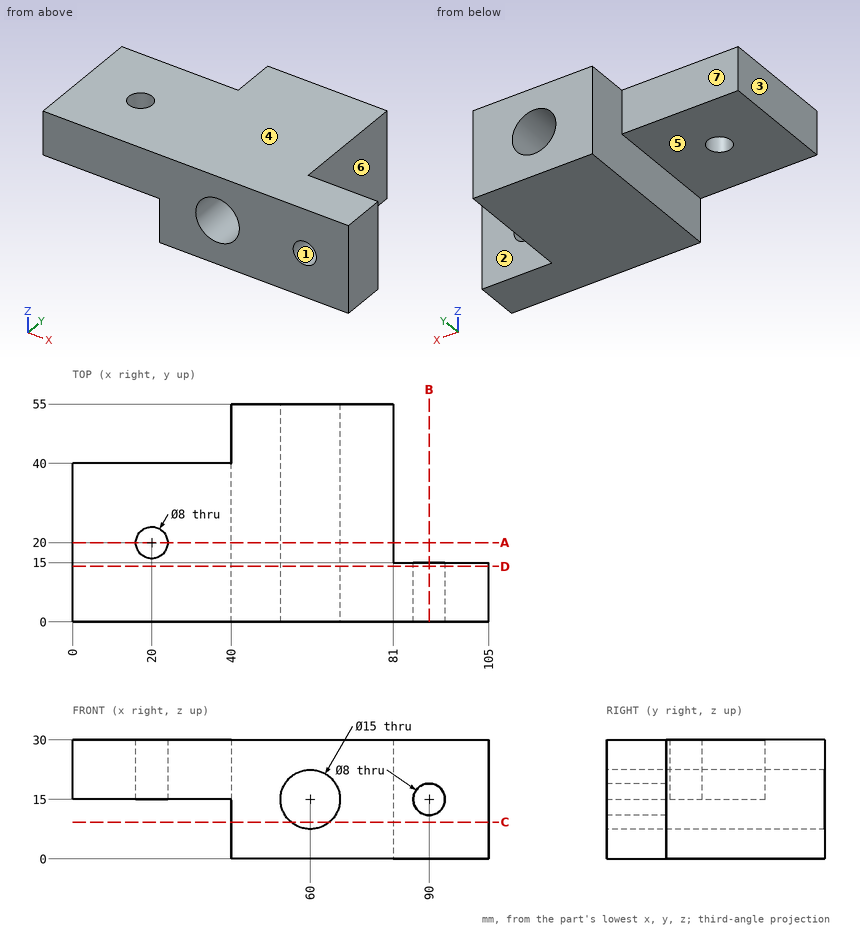
For this review, use the dimensioned drawing (mm, ordinates from the lowest corner) and the shaded views. A direction names the side the tool comes from. Round coordinates to 2 decimals unless told otherwise and drop trailing zeros. Write each loop counter-clockwise with the first axis right and the second up, starting at its lowest first coordinate (ties: lowest second). Pieces come first, ordered by that corner, then holes. Notation, with made-up numbers: (-26.75, -2) - (23.25, -2) arc R26 cw to (23.25, 31) - close; hole circle Ø4 at (-32, 1.25). An arc over 180 degrees is marked (long way). One line per item, written item: value. Start each with the question number.
1. Clearance check with flat-ended pins moving along their axes: P1, Ø16.5, axis at x = 20, z = 24, coming from the +Y side; P2, Ø2, axis at y = 44.5, z = 21, coming from the +X side; P3, Ø20, axis at x = 10.5, y = 16.5, coming from the -Z side; P4, Ø4, axis at x = 34, z = 12, coming from the -Y side. State where each tip first meets the part, or that it passes through.
2. Consider section B-B on x = 90. Write out the cut boundary in (y, z), and give its area (3 significant figures).
3. To check wall thickness, follow L1, parallel to Z at x = 90, y = 6.75; L2, parallel to Z at x = 60, y = 35; L3, parallel to X at y = 14, z = 13. State the ranges of each line that lie inside material, in increasing order. Write a range as from..to.
4. Consider section C-C on z = 9.25. Write out the cut boundary in (x, y).
5. Consider section A-A on y = 20. Write out the cut boundary in (x, z).
6. Consider section D-D on y = 14. Write out the cut boundary in (x, z).
7. The part is to be moulded in two halves that separate along X. For the marked faces 1, 2 and 3, say which applies: released by +X, released by -X, zero draft, split by the parting line, or undercut.
8. Machinability: for the marked faces 4, 5, 6 and 7, which of the approach directions +Z, -Z, +X, -X, +Y, -Y give a long, thin tool a straight path to every point of the face, cutting with its end or side? Answer none if there is none.
Checks:
1. P1: stops at y = 40
1. P2: stops at x = 81
1. P3: stops at z = 15
1. P4: passes through
2. outline: (0, 0) - (15, 0) - (15, 11) - (0, 11) - close; (0, 19) - (15, 19) - (15, 30) - (0, 30) - close
2. area: 330 mm^2
3. L1: z = 0..11, 19..30
3. L2: z = 0..7.5, 22.5..30
3. L3: x = 40..52.77, 67.23..86.54, 93.46..105
4. outline: (40, 0) - (55.18, 0) - (55.18, 55) - (40, 55) - close; (64.82, 0) - (105, 0) - (105, 15) - (81, 15) - (81, 55) - (64.82, 55) - close
5. outline: (0, 15) - (16, 15) - (16, 30) - (0, 30) - close; (24, 15) - (40, 15) - (40, 0) - (81, 0) - (81, 30) - (24, 30) - close; hole circle Ø15 at (60, 15)
6. outline: (0, 15) - (40, 15) - (40, 0) - (105, 0) - (105, 30) - (0, 30) - close; hole circle Ø15 at (60, 15); hole circle Ø8 at (90, 15)
7. face 1: undercut
7. face 2: zero draft
7. face 3: released by -X
8. face 4: +Z, +X, -X, +Y, -Y
8. face 5: -Z, -X, +Y, -Y
8. face 6: +Z, -Z, +X, +Y
8. face 7: +Z, -Z, -X, +Y
